For this review, use the dimensioned drawing (mm, ordinates from the lowest corner) and the shaded views. A direction names the side the tool comes from. Round coordinates to 2 decimals unless told otherwise and drop trailing zeros. Write each loop counter-clockwise with the first axis right and the second up, starting at its lowest first coordinate (ties: lowest second). Pieces come first, ordered by that corner, then holes. Notation, with made-up numbers: M 78,-36 L 134,-36 A23 ccw 134,-7 Z; hole C -39,44 d8. An arc over 180 degrees is marked long. Answer in a Markdown table with one row per item.
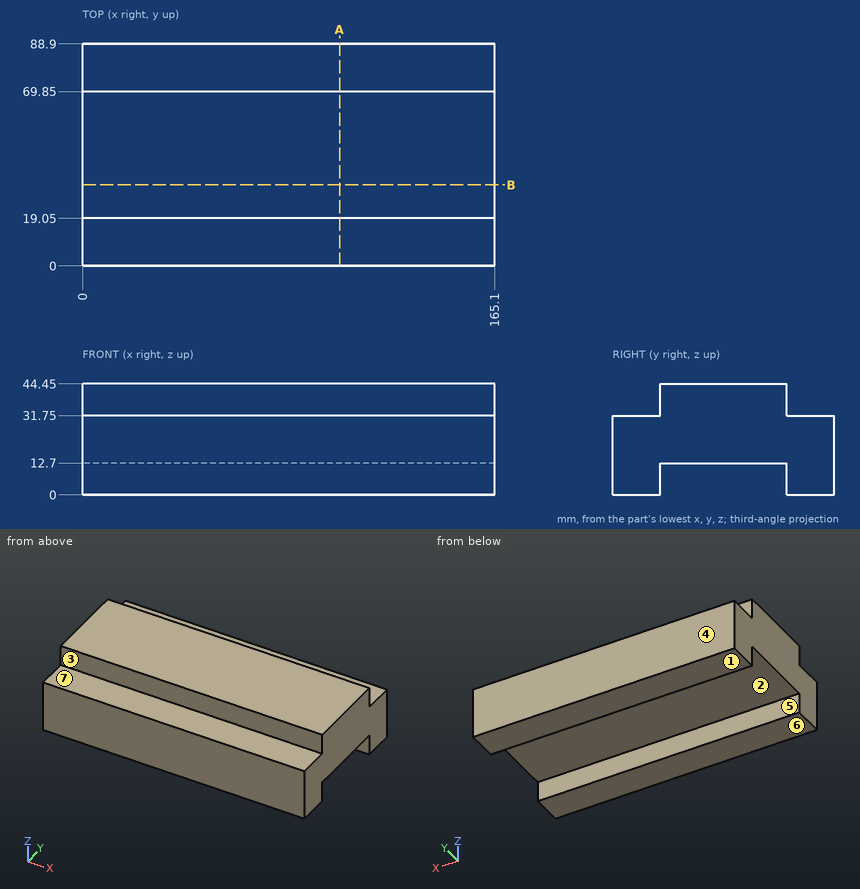
Q1. Take a section at B-B (y = 32.5). State the section outline as (x, z) points, then the cut area to 3 significant figures.
Found:
| item | result |
|---|---|
| outline | M 0,12.7 L 165.1,12.7 L 165.1,44.45 L 0,44.45 Z |
| area | 5,240 mm² |
Q2. For probe 1 along Y at (x, z) = (42.5, 12); probe 2 along Z at (x, y) = (143.5, 25.5); probe 3 along Y at (x, z) = (87, 39), list the stretches that pass through material, from the lowest coordinate up.
Found:
| item | result |
|---|---|
| probe 1 | 0 to 19.05, 69.85 to 88.9 |
| probe 2 | 12.7 to 44.45 |
| probe 3 | 19.05 to 69.85 |
Q3. Machinability: for the marked faces 5, 6 and 7, which of the approach directions +Z, -Z, +X, -X, +Y, -Y give a long, thin tool a straight path to every point of the face, cutting with its end or side? Answer none if there is none.
Found:
| item | result |
|---|---|
| face 5 | -Z, +X, -X |
| face 6 | -Z, +X, -X, +Y, -Y |
| face 7 | +Z, +X, -X, -Y |
Q4. Insertion check: P1, Ø5.5, axis at x = 99.5, y = 76, coming from the +Z side; P2, Ø6, axis at x = 68.5, z = 36.5, coming from the -Y side; P3, Ø4, axis at x = 82, z = 37.5, coming from the +Y side. Each pin has a flat end and moves straight along its axis. Give the tip position at first contact, or say it passes through.
Found:
| item | result |
|---|---|
| P1 | z = 31.75 |
| P2 | y = 19.05 |
| P3 | y = 69.85 |
Q5. Mouldability with a two-part tool opening along Y and no side actions: class the marked faces 1, 2, 3 and 4 as +Y half, -Y half, draft (parallel to the pull), parting line (faces both ways), or undercut.
Found:
| item | result |
|---|---|
| face 1 | draft |
| face 2 | undercut |
| face 3 | -Y half |
| face 4 | +Y half |
Q6. Take a section at A-A (x = 103). State the section outline as (y, z) points, then the cut area to 3 significant figures.
Found:
| item | result |
|---|---|
| outline | M 0,0 L 19.05,0 L 19.05,12.7 L 69.85,12.7 L 69.85,0 L 88.9,0 L 88.9,31.75 L 69.85,31.75 L 69.85,44.45 L 19.05,44.45 L 19.05,31.75 L 0,31.75 Z |
| area | 2,820 mm² |
